from build123d import *

# Parameters (mm, degrees)
F0_R     = 25.4
F1_DEPTH = 76.2
F2_R     = 12.7
F3_DEPTH = 105.41
F4_R     = 3.8838784961
F5_DEPTH = 133.35
F6_R     = 4.6082025667
F7_DEPTH = 145.542


# Not quite as in the source:
# - a fillet or chamfer that OpenCascade refuses, or shapes differently, is made with other operations: its cross-section is extruded or revolved along the edge and cut away or added


with BuildPart() as f1:
    # F0 (on Front) → F1 (new body)
    with BuildSketch(Plane.XZ):
        Circle(F0_R)
    extrude(amount=F1_DEPTH)

    # F2 (on face) → F3 (cut)
    with BuildSketch(Plane.XZ.offset(76.2)):
        Circle(F2_R)
    extrude(amount=-F3_DEPTH, mode=Mode.SUBTRACT)

    # F4 (on Front) → F5 (cut)
    with BuildSketch(Plane.XZ):
        with Locations((-19.7816453874, 11.8296807632)):
            Circle(F4_R)
    extrude(amount=F5_DEPTH, mode=Mode.SUBTRACT)

    # F6 (on Front) → F7 (cut)
    with BuildSketch(Plane.XZ):
        with Locations((-7.7014984563, 17.5422988832)):
            Circle(F6_R)
    extrude(amount=F7_DEPTH, mode=Mode.SUBTRACT)

    # F8: fillet of radius 5.08 on 2 edges, made by hand

    # F8_s1 → F8_t2 (revolve, cut)
    with BuildSketch(Plane.XY):
        with BuildLine():
            ThreePointArc((17.78, -76.2), (14.1878975516, -74.7121024484), (12.7, -71.12))
            Line((12.7, -71.12), (12.7, -76.2))
            Line((12.7, -76.2), (17.78, -76.2))
        make_face()
    revolve(axis=Axis((0, -76.2, 0), (0, -1, 0)), mode=Mode.SUBTRACT)

    # F8_s3 → F8_t4 (revolve, cut)
    with BuildSketch(Plane.XY.offset(17.5422988832)):
        with BuildLine():
            ThreePointArc((1.9867041104, -76.2), (-1.605398338, -74.7121024484), (-3.0932958896, -71.12))
            Line((-3.0932958896, -71.12), (-3.0932958896, -76.2))
            Line((-3.0932958896, -76.2), (1.9867041104, -76.2))
        make_face()
    revolve(axis=Axis((-7.7014984563, -76.2, 17.5422988832), (0, 1, 0)), mode=Mode.SUBTRACT)

    # F9: fillet of radius 5.08 on 2 edges, made by hand

    # F9_s1 → F9_t2 (revolve, cut)
    with BuildSketch(Plane.XY):
        with BuildLine():
            ThreePointArc((17.7809656854, 0.0004), (14.1878975516, -1.4878975516), (12.6996, -5.0809656854))
            Line((12.6996, -5.0809656854), (12.1914634315, -5.0809656854))
            ThreePointArc((12.1914634315, -5.0809656854), (12.1918634315, -2.5404828427), (12.1918634315, 0))
            Line((12.1918634315, 0), (12.7, 0.5081365685))
            ThreePointArc((12.7, 0.5081365685), (15.2404828427, 0.5081365685), (17.7809656854, 0.5085365685))
            Line((17.7809656854, 0.5085365685), (17.7809656854, 0.0004))
        make_face()
    revolve(axis=Axis((0, 0, 0), (0, -1, 0)), mode=Mode.SUBTRACT)

    # F9_s3 → F9_t4 (revolve, cut)
    with BuildSketch(Plane.XY.offset(17.5422988832)):
        with BuildLine():
            ThreePointArc((1.9876697958, 0.0004), (-1.605398338, -1.4878975516), (-3.0936958896, -5.0809656854))
            Line((-3.0936958896, -5.0809656854), (-3.6018324581, -5.0809656854))
            ThreePointArc((-3.6018324581, -5.0809656854), (-3.6014324581, -2.5404828427), (-3.6014324581, 0))
            Line((-3.6014324581, 0), (-3.0932958896, 0.5081365685))
            ThreePointArc((-3.0932958896, 0.5081365685), (-0.5528130469, 0.5081365685), (1.9876697958, 0.5085365685))
            Line((1.9876697958, 0.5085365685), (1.9876697958, 0.0004))
        make_face()
    revolve(axis=Axis((-7.7014984563, 0, 17.5422988832), (0, -1, 0)), mode=Mode.SUBTRACT)


solid = f1.part
Here's how the part is built. I have some questions about the finished solid (model axes, mm). Coordinates: 2 decimals unless noted, no trailing zeros. Order: outer loops, then holes, each group sorted by start corner. A loop starts at its lowest first (then second) coordinate and runs counter-clockwise, first axis right, second up. Notation, with made-up numbers: M -12.5,-17 L 42.5,-17 A21 cw 42.5,10 Z; hole C -24,36 d2. An arc over 180 degrees is marked long. Answer as CSV lines item,"result".
Item 1: Imagine slicing it at A-A on z = 0. Write out the boundary of the cut face in (x, y), plus the area to 3 significant figures.
Results found:
outline,"M -25.4,-76.2 L -17.78,-76.2 A5.08 ccw -12.7,-71.12 L -12.7,-5.02 A5.08 ccw -17.72,0 L -25.4,0 Z; M 12.7,-71.12 A5.08 ccw 17.78,-76.2 L 25.4,-76.2 L 25.4,0 L 17.72,0 A5.08 ccw 12.7,-5.02 Z"
area,"1,910 mm2"
Item 2: Imagine slicing it at B-B on y = -52. Write out the boundary of the cut face in (x, z), plus the area to 3 significant figures.
Results found:
outline,"M -23.28,10.15 A25.4 ccw long -19.96,15.71 A3.88 cw long Z; hole C 0,0 d25.4; hole C -7.7,17.54 d9.22"
area,"1,410 mm2"
Item 3: Imagine slicing it at C-C on x = -7. Give the number of separate pieces and of enclosed holes in the cut face, plus the area to 3 significant figures.
Results found:
separate pieces,"3"
enclosed holes,"0"
area,"1,380 mm2"
Item 4: For pin 1 (8 mm diameter, centred on x = 19.5, y = -53.5, fed in from -Z); pin 2 (10.5 mm diameter, centred on x = -7.7, z = 17.54, fed in from +Y); pin 3 (2 mm diameter, centred on x = 1.5, z = 14, fed in from +Y), each with a flat end and sliding along its axis, tell me the tip position at first contact or that it passes through.
Results found:
pin 1,"z = -20.12"
pin 2,"y = -2.6"
pin 3,"y = -0.78"
Item 5: We'd pull the mould along X, two halves only. Please class faces 1 (the face through (21.23, -37.567, -13.944)), 2 (the face through (-2.75, -38.53, -12.4)), 3 (the face through (7, -76.2, -17)): +X half, -X half, draft (parallel to the pull), parting line (faces both ways), or undercut.
Results found:
face 1,"parting line"
face 2,"undercut"
face 3,"draft"
Item 6: Imagine slicing it at D-D on x = 21.5. Write out the boundary of the cut face in (y, z).
Results found:
outline,"M -76.2,-13.52 L 0,-13.52 L 0,13.52 L -76.2,13.52 Z"
Item 7: If I drill on line 1 (Z direction, x = 0, y = -48.5); line 2 (X direction, y = -38.5, z = 5.5), over which ranges is the centre line in solid material (lowest first)?
Results found:
line 1,"-25.4 to -12.7, 12.7 to 25.4"
line 2,"-24.8 to -11.45, 11.45 to 24.8"
